Here's how the part is built. I have some questions about the finished solid (model axes, mm). A direction names the side the tool comes from. Coordinates: 2 decimals unless noted, no trailing zeros. Loops run counter-clockwise (first coordinate to the right, second up) from the corner with the lowest first, then second, coordinate; pieces in that order, holes last. Notation, with made-up numbers: (-22.5, 54) -> (9.5, 54) arc R18 cw to (9.5, 88) -> close; hole circle Ø3 at (33, -28). An arc over 180 degrees is marked (long way). Answer as a JSON object with one key per item and string values. Group by question number.
1) I need wall thicknesses on probe 1 along Z at (x, y) = (28, 50); probe 2 along Y at (x, z) = (46, 45.5). Which ranges of each line are inside material? Lowest first, please. Write a range as [from, to].
2) I want a section at C-C (y = 9.5). Write out the boundary of the cut face in (x, z).
3) I'm going to push flat-ended pins straight in: pin 1 (9 mm diameter, centred on x = 32.5, y = 25.5, fed in from +Z); pin 2 (2.5 mm diameter, centred on y = 21.16, z = 53, fed in from +X); pin 3 (1.5 mm diameter, centred on x = 37.5, y = 15.5, fed in from -Z); pin 4 (12 mm diameter, centred on x = 23.5, z = 9.5, fed in from +Y). Where does each tip first touch, or does it pass through?
4) I want a section at D-D (z = -3). Write out the boundary of the cut face in (x, y).
5) I want a section at B-B (x = 33). Write out the boundary of the cut face in (y, z).
6) I want a section at A-A (z = 32.5). Write out the boundary of the cut face in (x, y).
7) Which directions (+Z, -Z, +X, -X, +Y, -Y) give clear straight access to the entire face, cutting with the end or side of a thin tool? Please do faces 4 (the flat face through (32.151, 3, 25)), 5 (the cylindrical face through (43.724, 2.425, 49.43)), 6 (the flat face through (43.007, 17.771, 5.371)).
8) If we mould it in two halves opening along Z, with no side actions, what happens to faces 1 (the flat face through (43.007, 17.771, 44.629)), 2 (the flat face through (57, 24, 56)), 3 (the flat face through (27.436, 9.538, 1.855))? For each: +Z half, -Z half, draft (parallel to the pull), parting line (faces both ways), or undercut.
```python
from build123d import *

# Parameters (mm, degrees)
EXTRUDE_1_DEPTH     = 50
EXTRUDE_3_DEPTH     = 33.199998
EXTRUDE_4_REACH     = 79.048
SKETCH_4_W          = 50
SKETCH_4_H          = 2.121320344
CUT_EXTRUDE_1_DEPTH = 99.405896905
SKETCH_8_W          = 62
SKETCH_8_H          = 44.689148571
SKETCH_8_R          = 1.5
EXTRUDE_5_DEPTH     = 3
FILLET_1_R          = 10
FILLET_2_R          = 2


with BuildPart() as part:
    # 草图1 → 凸台-拉伸1 (new body)
    with BuildSketch(Plane.XY):
        Polygon((25.716046069, 61.209761814), (43.929249505, 61.209761814), (58.626662914, 46.512348406), (58.626662914, 1.823199835), (32.150717778, 1.823199835), (32.150717778, 4.823199835), (55.626662914, 28.29914497), (25.716046069, 58.209761814), align=None)
    extrude(amount=EXTRUDE_1_DEPTH)

    # 草图3 → 凸台-拉伸3 (add)
    with BuildSketch(Plane(origin=(41.962903942, 41.962903942, 0), x_dir=(0, 0, 1), z_dir=(-0.7071067811865476, -0.7071067811865476, 0))):
        Polygon((50, -19.323473251), (46.15, -19.323473251), (43.15, -19.323473251), (46.15, -16.323473251), (46.15, 19.976526749), (43.15, 22.976526749), (46.15, 22.976526749), (50, 22.976526749), align=None)
        Polygon((0, 22.976526749), (0, -19.323473251), (3.85, -19.323473251), (6.85, -19.323473251), (3.85, -16.323473251), (3.85, 19.976526749), (6.85, 22.976526749), (3.85, 22.976526749), align=None)
    extrude(amount=EXTRUDE_3_DEPTH)

    # 凸台-拉伸4: up to this plane
    extrude_4_end = Plane(origin=(25.716046069, 61.209761814, 50), z_dir=(0, -1, 0))
    # 草图4 → 凸台-拉伸4 (add, up to the surface)
    with BuildSketch(Plane(origin=(18.486958806, 18.486958806, 0), x_dir=(0, 0, 1), z_dir=(-0.7071067811865477, -0.7071067811865475, 0)), mode=Mode.PRIVATE) as extrude_4_sk1:
        with Locations((25, 24.037186921)):
            Rectangle(SKETCH_4_W, SKETCH_4_H)
    extrude_4_tool1 = split(extrude(extrude_4_sk1.sketch, amount=-EXTRUDE_4_REACH, mode=Mode.PRIVATE), bisect_by=extrude_4_end, keep=Keep.BOTH, mode=Mode.PRIVATE)
    add(extrude_4_tool1.solids().sort_by_distance((1.490101, 35.483817, 25))[0])

    # 草图5 → 切除-拉伸1 (cut, through all)
    with BuildSketch(Plane(origin=(0, 0, 0), x_dir=(-1, 0, 0), z_dir=(0, 0, -1))):
        Polygon((-35.014500242, 48.911307642), (-46.328208741, 37.597599143), (-22.852263606, 14.121654007), (-11.538555107, 25.435362506), align=None)
    extrude(amount=-CUT_EXTRUDE_1_DEPTH, mode=Mode.SUBTRACT)

    # 草图8 → 凸台-拉伸5 (add)
    with BuildSketch(Plane(origin=(58.626662914, 0, 0), x_dir=(0, 0, -1), z_dir=(1, 0, 0))):
        with Locations((-25, 24.16777412)):
            Rectangle(SKETCH_8_W, SKETCH_8_H)
        with Locations(Location((-53, 39.162348406, 0), (0, 0, 90))):
            Circle(SKETCH_8_R, mode=Mode.SUBTRACT)
        with Locations(Location((-53, 33.162348406, 0), (0, 0, 90))):
            Circle(SKETCH_8_R, mode=Mode.SUBTRACT)
        with Locations(Location((-53, 27.162348406, 0), (0, 0, 90))):
            Circle(SKETCH_8_R, mode=Mode.SUBTRACT)
        with Locations(Location((-53, 21.162348406, 0), (0, 0, 90))):
            Circle(SKETCH_8_R, mode=Mode.SUBTRACT)
        with Locations(Location((-53, 15.162348406, 0), (0, 0, 90))):
            Circle(SKETCH_8_R, mode=Mode.SUBTRACT)
        with Locations(Location((-53, 9.162348406, 0), (0, 0, 90))):
            Circle(SKETCH_8_R, mode=Mode.SUBTRACT)
        with Locations(Location((3, 9.162348406, 0), (0, 0, 270))):
            Circle(SKETCH_8_R, mode=Mode.SUBTRACT)
        with Locations(Location((3, 15.162348406, 0), (0, 0, 270))):
            Circle(SKETCH_8_R, mode=Mode.SUBTRACT)
        with Locations(Location((3, 21.162348406, 0), (0, 0, 270))):
            Circle(SKETCH_8_R, mode=Mode.SUBTRACT)
        with Locations(Location((3, 27.162348406, 0), (0, 0, 270))):
            Circle(SKETCH_8_R, mode=Mode.SUBTRACT)
        with Locations(Location((3, 33.162348406, 0), (0, 0, 270))):
            Circle(SKETCH_8_R, mode=Mode.SUBTRACT)
        with Locations(Location((3, 39.162348406, 0), (0, 0, 270))):
            Circle(SKETCH_8_R, mode=Mode.SUBTRACT)
    extrude(amount=-EXTRUDE_5_DEPTH)

    # 圆角1
    fillet_1_edges = [part.edges().sort_by_distance(p)[0] for p in [
        (25.716046069, 61.209761814, 25),
        (43.929249505, 61.209761814, 25),
    ]]
    fillet(fillet_1_edges, radius=FILLET_1_R)

    # 圆角2
    fillet_2_edges = [part.edges().sort_by_distance(p)[0] for p in [
        (52.742422303, 52.396589016, 0),
        (57.126662914, 1.823199835, -6),
        (57.126662914, 1.823199835, 56),
        (57.126662914, 46.512348406, 56),
        (57.126662914, 46.512348406, -6),
        (34.822647787, 61.209761814, 0),
        (34.822647787, 61.209761814, 50),
        (11.763607408, 47.257323152, 0),
        (26.031347369, 60.448557139, 0),
        (43.613948205, 60.448557139, 0),
        (11.763607408, 47.257323152, 50),
        (26.031347369, 60.448557139, 50),
        (43.613948205, 60.448557139, 50),
        (43.888690346, 1.823199835, 50),
        (43.888690346, 1.823199835, 0),
        (52.742422303, 52.396589016, 50),
    ]]
    fillet(fillet_2_edges, radius=FILLET_2_R)


solid = part.part
```
Determined:
{
 "1": {"probe 1": "[0, 3.85], [46.15, 50]", "probe 2": "[1.82, 22], [37.93, 59.05]"},
 "2": {"outline": "(27.47, 0) -> (55.63, 0) -> (55.63, -1.54) -> (58.63, -1.54) -> (58.63, 51.54) -> (55.63, 51.54) -> (55.63, 50) -> (27.47, 50) -> (27.47, 46.15) -> (32.58, 46.15) -> (36.83, 43.15) -> (36.83, 6.85) -> (32.58, 3.85) -> (27.47, 3.85) -> close; (55.63, -6) -> (58.63, -6) -> (58.63, -4.46) -> (55.63, -4.46) -> close; (55.63, 54.46) -> (58.63, 54.46) -> (58.63, 56) -> (55.63, 56) -> close"},
 "3": {"pin 1": "z = 50", "pin 2": "through", "pin 3": "z = 0", "pin 4": "y = 61.2"},
 "4": {"outline": "(55.63, 1.82) -> (58.63, 1.82) -> (58.63, 7.66) -> (55.63, 7.66) -> close; (55.63, 10.66) -> (58.63, 10.66) -> (58.63, 13.66) -> (55.63, 13.66) -> close; (55.63, 16.66) -> (58.63, 16.66) -> (58.63, 19.66) -> (55.63, 19.66) -> close; (55.63, 22.66) -> (58.63, 22.66) -> (58.63, 25.66) -> (55.63, 25.66) -> close; (55.63, 28.66) -> (58.63, 28.66) -> (58.63, 31.66) -> (55.63, 31.66) -> close; (55.63, 34.66) -> (58.63, 34.66) -> (58.63, 37.66) -> (55.63, 37.66) -> close; (55.63, 40.66) -> (58.63, 40.66) -> (58.63, 46.51) -> (55.63, 46.51) -> close"},
 "5": {"outline": "(1.82, 2) arc R2 ccw to (3.82, 0) -> (24.27, 0) -> (24.27, 3.85) -> (9.92, 3.85) -> (5.67, 6.85) -> (5.67, 43.15) -> (9.92, 46.15) -> (24.27, 46.15) -> (24.27, 50) -> (3.82, 50) arc R2 ccw to (1.82, 48) -> close; (46.9, 0) -> (59.21, 0) arc R2 ccw to (61.21, 2) -> (61.21, 48) arc R2 ccw to (59.21, 50) -> (46.9, 50) -> (46.9, 46.15) -> (50.93, 46.15) -> (50.93, 3.85) -> (46.9, 3.85) -> close"},
 "6": {"outline": "(0.74, 36.23) -> (2.24, 34.73) -> (25.72, 58.21) -> (55.63, 28.3) -> (32.15, 4.82) -> (32.15, 1.82) -> (58.63, 1.82) -> (58.63, 46.51) -> (46.86, 58.28) arc R10 ccw to (39.79, 61.21) -> (29.86, 61.21) arc R10 ccw to (22.79, 58.28) -> close"},
 "7": {"face 4": "+Z, -Z, -X, -Y", "face 5": "+Z, -X, -Y", "face 6": "-X"},
 "8": {"face 1": "undercut", "face 2": "+Z half", "face 3": "draft"}
}
